Design review of the part built by this model. Coordinates are the model's own, in mm. Face numbers are marked on the shaded views. A direction names the side the tool comes from. Coordinates: 2 decimals unless noted, no trailing zeros. Loops run counter-clockwise (first coordinate to the right, second up) from the corner with the lowest first, then second, coordinate; pieces in that order, holes last. Notation, with made-up numbers: M 73,-7.5 L 106,-7.5 A6 ccw 106,2.5 Z; hole C 42,1.25 d11. An arc over 180 degrees is marked long. Write item = value, one per line. Start each with the question number.
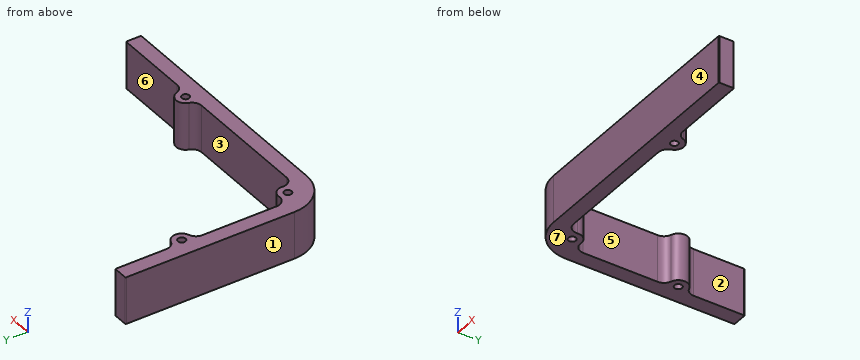
Autodesk Inventor part; units mm, degrees
ref_plane "YZ Plane" through (0, 0, 0) normal (1, 0, 0) x (0, 1, 0)
ref_plane "XZ Plane" through (0, 0, 0) normal (0, 1, 0) x (-1, 0, 0)
ref_plane "XY Plane" through (0, 0, 0) normal (0, 0, 1) x (1, 0, 0)
sketch "Sketch1" plane through (0, 0, 0) normal (0, 0, 1) x (1, 0, 0)
  line L0 (-74.8, 54.8) -> (74.8, 54.8)
  line L1 (74.8, 54.8) -> (74.8, -54.8)
  line L2 (74.8, -54.8) -> (-74.8, -54.8)
  line L3 (-74.8, -54.8) -> (-74.8, 54.8)
  line L4 (-74.8, 54.8) -> (74.8, -54.8) construction
  line L5 (74.8, 54.8) -> (-74.8, -54.8) construction
  line L6 (-66.8, 54.8) -> (-66.8, -46.8)
  line L7 (-66.8, -46.8) -> (74.8, -46.8)
  point P0 (0, 0)
  dimension "d0" = 149.6
  dimension "d1" = 109.6
  dimension "d2" = 8
  dimension "d3" = 8
extrude "Extrusion1" add sketch "Sketch1" along normal blind 25 contours L0 L6 L7 L1 L2 L3
fillet "Fillet1" radius 12 1 edges at (-66.8, -46.8, 12.5)
fillet "Fillet2" radius 20 1 edges at (-74.8, -54.8, 12.5)
sketch "Sketch2" plane through (0, 0, 25) normal (0, 0, 1) x (1, 0, 0)
  circle A0 centre (25.2, -44.8) radius 5
  circle A1 centre (-60.8, -40.8) radius 5
  circle A2 centre (-64.8, 18.2) radius 5
  line L0 (-54.8, -54.8) -> (74.8, -54.8)
  line L1 (-74.8, 54.8) -> (-74.8, -34.8)
  point P0 (0, 0)
  dimension "d8" = 10
  dimension "d9" = 10
  dimension "d10" = 14
  dimension "d11" = 14
  dimension "d12" = 73
  dimension "d13" = 100
  dimension "d14" = 10
extrude "Extrusion2" add sketch "Sketch2" against normal up to surface (25 mm away)
sketch "Sketch3" plane through (0, 0, 25) normal (0, 0, 1) x (1, 0, 0)
  arc A0 (-66.8, 13.6174) -> (-66.8, 22.7826) centre (-64.8, 18.2) ccw
  arc A1 (-59.8147, -45.702) -> (-65.702, -39.8147) centre (-60.8, -40.8) ccw
  arc A2 (29.7826, -46.8) -> (20.6174, -46.8) centre (25.2, -44.8) ccw
  point P0 (0, 0)
hole "Hole1" at (-64.8, 18.2, 25) at (-60.8, -40.8, 25) at (25.2, -44.8, 25) direction (0, 0, -1) diameter 4 end through all
fillet "Fillet3" radius 5 6 edges at (29.7826, -46.8, 12.5) (20.6174, -46.8, 12.5) (-65.702, -39.8147, 12.5) (-59.8147, -45.702, 12.5) (-66.8, 22.7826, 12.5) (-66.8, 13.6174, 12.5)
fillet "Fillet4" radius 0.4 4 edges at (-74.8, 54.8, 12.5) (-66.8, 54.8, 12.5) (74.8, -54.8, 12.5) (74.8, -46.8, 12.5)
equation "\"d3\" = d2"
equation "\"d9\" = d8"
equation "\"d11\" = d10"
properties part number "Corner"
(1) Mouldability with a two-part tool opening along Y and no side actions: class the marked faces 4, 5, 6 and 7 as +Y half, -Y half, draft (parallel to the pull), parting line (faces both ways), or undercut.
(2) To check wall thickness, follow L1, parallel to Y at x = -60.8, z = 15.25; L2, parallel to X at y = -40.8, z = 11.25; L3, parallel to X at y = 18.2, z = 11.75. State the ranges of each line that lie inside material, in increasing order.
(3) Insertion check: pin 1 (1.5 mm diameter, centred on x = -49.5, z = 11.5, fed in from +Y); pin 2 (7.5 mm diameter, centred on y = 34.5, z = 6.5, fed in from +X). Each pin has a flat end and moves straight along its axis. Give the tip position at first contact, or say it passes through.
(4) Take a section at A-A (y = 18.2). State the section outline as (x, z) points.
(5) Tool access review of the marked faces 1, 2 and 3: name each direction out of +Z, -Z, +X, -X, +Y, -Y from which nothing blocks a thin tool from reaching the whole face with its end or side.
(6) Take a section at B-B (x = -64.8). Give the number of separate pieces and of enclosed holes in the cut face, plus the area to 3 significant figures.
(7) Take a section at D-D (x = 43). State the section outline as (y, z) points.
Results list:
q1.face_4 = -Y half
q1.face_5 = undercut
q1.face_6 = +Y half
q1.face_7 = draft
q2.L1 = -53.88 to -42.8, -38.8 to -35.8, 15.2 to 21.2
q2.L2 = -73.88 to -62.8, -58.8 to -55.8, 22.2 to 28.2
q2.L3 = -74.8 to -66.8, -62.8 to -59.8
q3.pin_1 = -46.8
q3.pin_2 = -66.8
q4.outline = M -74.8,0 L -66.8,0 L -66.8,25 L -74.8,25 Z; M -62.8,0 L -59.8,0 L -59.8,25 L -62.8,25 Z
q5.face_1 = +Z, -Z, -X, +Y, -Y
q5.face_2 = +Z, -Z, +X, +Y
q5.face_3 = +Z, -Z, +Y
q6.separate_pieces = 3
q6.enclosed_holes = 0
q6.area = 609 mm^2
q7.outline = M -54.8,0 L -46.8,0 L -46.8,25 L -54.8,25 Z
